Part model, mm, in its own coordinate system. Round coordinates to 2 decimals unless told otherwise and drop trailing zeros. Loops run counter-clockwise (first coordinate to the right, second up) from the corner with the lowest first, then second, coordinate; pieces in that order, holes last.
from build123d import *

# Parameters (mm, degrees)
EXTRUDE_1_DEPTH     = 1
SKETCH_2_W          = 2.2
SKETCH_2_H          = 2.4
SKETCH_2_H_2        = 12.6
CUT_EXTRUDE_1_DEPTH = 81.802227692
SKETCH_4_R          = 1.35
CUT_EXTRUDE_3_DEPTH = 81.802227692
FILLET_1_R          = 10
FILLET_2_R          = 2


with BuildPart() as part:
    # Sketch 1 → Extrude 1 (new, symmetric)
    with BuildSketch(Plane.XY):
        Polygon((15, 30), (-15, 30), (-75, 10), (-75, 0), (75, 0), (75, 10), align=None)
    extrude(amount=EXTRUDE_1_DEPTH, both=True)

    # Sketch 2 → Cut-Extrude 1 (cut, through all)
    with BuildSketch(Plane.XY.offset(1)):
        with BuildLine():
            Line((-1.1, 12.6), (-1.1, 15))
            ThreePointArc((-1.1, 15), (-2.3, 13.8), (-1.1, 12.6))
        make_face()
        with Locations((0, 13.8)):
            Rectangle(SKETCH_2_W, SKETCH_2_H)
        with BuildLine():
            ThreePointArc((1.1, 12.6), (2.3, 13.8), (1.1, 15))
            Line((1.1, 15), (1.1, 12.6))
        make_face()
        with Locations((0, 6.3)):
            Rectangle(SKETCH_2_W, SKETCH_2_H_2)
    extrude(amount=-CUT_EXTRUDE_1_DEPTH, mode=Mode.SUBTRACT)

    # Sketch 4 → Cut-Extrude 3 (cut, through all)
    with BuildSketch(Plane.XY.offset(1)):
        with Locations((-12, 4)):
            Circle(SKETCH_4_R)
        with Locations(Location((12, 4, 0), (0, 0, 180))):
            Circle(SKETCH_4_R)
    extrude(amount=-CUT_EXTRUDE_3_DEPTH, mode=Mode.SUBTRACT)

    # Fillet 1
    fillet_1_edges = [part.edges().sort_by_distance(p)[0] for p in [
        (75, 10, 0),
        (-75, 10, 0),
    ]]
    fillet(fillet_1_edges, radius=FILLET_1_R)

    # Fillet 2
    fillet_2_edges = [part.edges().sort_by_distance(p)[0] for p in [
        (-15, 30, 0),
        (15, 30, 0),
        (75, 0, 0),
        (-75, 0, 0),
        (1.1, 0, 0),
        (-1.1, 0, 0),
    ]]
    fillet(fillet_2_edges, radius=FILLET_2_R)


solid = part.part
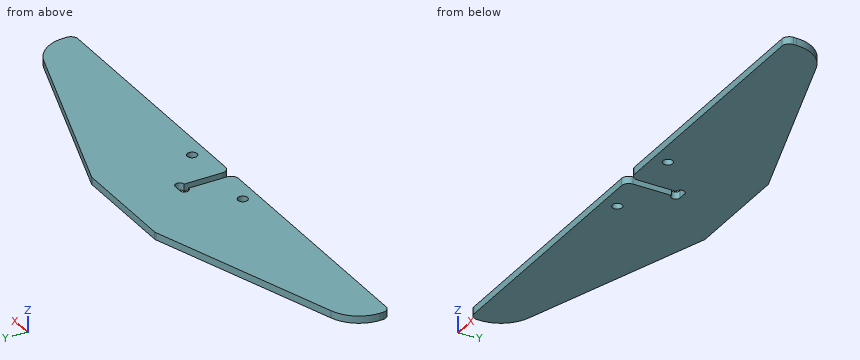
1) Slice it at B-B, the plane y = 8. Give the cut face in (x, z).
Values:
outline: (-73.54, -1) - (-1.1, -1) - (-1.1, 1) - (-73.54, 1) - close; (1.1, -1) - (73.54, -1) - (73.54, 1) - (1.1, 1) - close
2) Slice it at D-D, the plane x = 36. Give the cut face in (y, z).
Values:
outline: (0, -1) - (23, -1) - (23, 1) - (0, 1) - close
3) Slice it at A-A, the plane x = 12. Give the cut face in (y, z), then the cut area to 3 significant figures.
Values:
outline: (0, -1) - (2.65, -1) - (2.65, 1) - (0, 1) - close; (5.35, -1) - (30, -1) - (30, 1) - (5.35, 1) - close
area: 54.6 mm2
4) Wall check: line 1 along X through (y, z) = (2, 0); line 2 along Y through (x, z) = (12, -0.3); line 3 along X through (y, z) = (5, -0.8). Give the ranges that are in metal, low to high.
Values:
line 1: x = -75 to -1.1, 1.1 to 75
line 2: y = 0 to 2.65, 5.35 to 30
line 3: x = -74.75 to -12.91, -11.09 to -1.1, 1.1 to 11.09, 12.91 to 74.75
5) Slice it at C-C, the plane z = -0.15. Give the cut face in (x, y), then the cut area to 3 significant figures.
Values:
outline: (-75, 2) arc R2 ccw to (-73, 0) - (-3.1, 0) arc R2 ccw to (-1.1, 2) - (-1.1, 12.6) arc R1.2 cw to (-1.1, 15) - (1.1, 15) arc R1.2 cw to (1.1, 12.6) - (1.1, 2) arc R2 ccw to (3.1, 0) - (73, 0) arc R2 ccw to (75, 2) - (75, 2.79) arc R10 ccw to (68.16, 12.28) - (15.31, 29.9) arc R2 ccw to (14.68, 30) - (-14.68, 30) arc R2 ccw to (-15.31, 29.9) - (-68.16, 12.28) arc R10 ccw to (-75, 2.79) - close; hole circle Ø2.7 at (-12, 4); hole circle Ø2.7 at (12, 4)
area: 3,230 mm2
